Check sheet for the drawn part. Datum: minimum x, y, z corner. Units: mm. Coordinates: 2 decimals unless noted, no trailing zeros. Write each loop counter-clockwise with the first axis right and the second up, starting at its lowest first coordinate (ties: lowest second). Pieces come first, ordered by that corner, then holes. Notation, with made-up numbers: (-2.75, 44.5) - (6.25, 44.5) arc R9 ccw to (6.25, 57.5) - close; hole circle Ø2 at (39, 5.25). An arc over 180 degrees is marked (long way). Write each question's results on one line, items separated by ' | '.
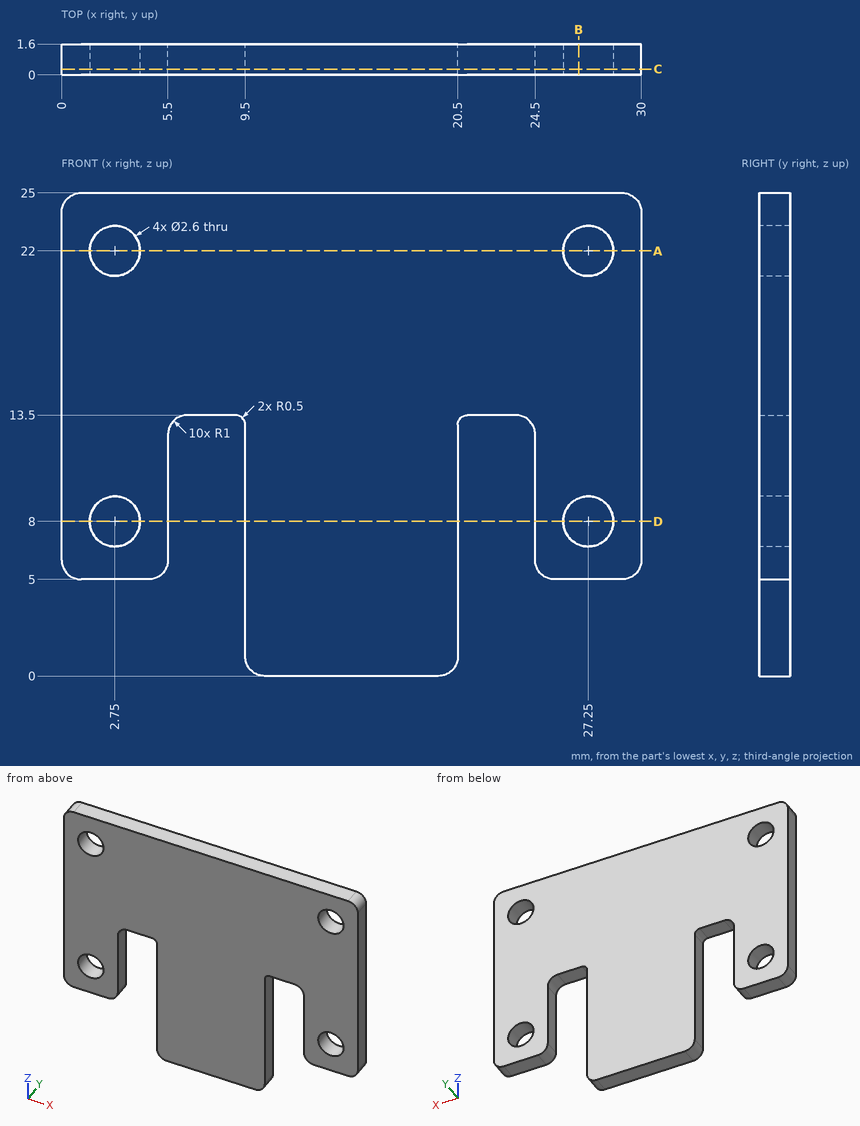
1. Sectioned sample at B-B (x = 26.75). Record the cut outline in (y, z).
Values follow:
outline: (0, 5) - (1.6, 5) - (1.6, 6.8) - (0, 6.8) - close; (0, 9.2) - (1.6, 9.2) - (1.6, 20.8) - (0, 20.8) - close; (0, 23.2) - (1.6, 23.2) - (1.6, 25) - (0, 25) - close
2. Sectioned sample at D-D (z = 8). Record the cut outline in (x, y), then the cut area to 3 significant figures.
Values follow:
outline: (0, 0) - (1.45, 0) - (1.45, 1.6) - (0, 1.6) - close; (4.05, 0) - (5.5, 0) - (5.5, 1.6) - (4.05, 1.6) - close; (9.5, 0) - (20.5, 0) - (20.5, 1.6) - (9.5, 1.6) - close; (24.5, 0) - (25.95, 0) - (25.95, 1.6) - (24.5, 1.6) - close; (28.55, 0) - (30, 0) - (30, 1.6) - (28.55, 1.6) - close | area: 26.9 mm^2
3. Sectioned sample at C-C (y = 0.3). Record the cut outline in (x, z), then the cut area to 3 significant figures.
Values follow:
outline: (0, 6) arc R1 ccw to (1, 5) - (4.5, 5) arc R1 ccw to (5.5, 6) - (5.5, 12.5) arc R1 cw to (6.5, 13.5) - (9, 13.5) arc R0.5 cw to (9.5, 13) - (9.5, 1) arc R1 ccw to (10.5, 0) - (19.5, 0) arc R1 ccw to (20.5, 1) - (20.5, 13) arc R0.5 cw to (21, 13.5) - (23.5, 13.5) arc R1 cw to (24.5, 12.5) - (24.5, 6) arc R1 ccw to (25.5, 5) - (29, 5) arc R1 ccw to (30, 6) - (30, 24) arc R1 ccw to (29, 25) - (1, 25) arc R1 ccw to (0, 24) - close; hole circle Ø2.6 at (2.75, 8); hole circle Ø2.6 at (2.75, 22); hole circle Ø2.6 at (27.25, 8); hole circle Ø2.6 at (27.25, 22) | area: 565 mm^2
4. Go/stop test with flat-tipped pins: pin 1 (3.5 mm diameter, centred on x = 2.75, z = 22, fed in from -Y); pin 2 (2.5 mm diameter, centred on x = 27.25, z = 8, fed in from -Y); pin 3 (0.8 mm diameter, centred on x = 22, y = 1, fed in from -Z). Record where each tip stops, or that it passes through.
Values follow:
pin 1: stops at y = 0 | pin 2: passes through | pin 3: stops at z = 13.5
5. Sectioned sample at A-A (z = 22). Record the cut outline in (x, y), then the cut area to 3 significant figures.
Values follow:
outline: (0, 0) - (1.45, 0) - (1.45, 1.6) - (0, 1.6) - close; (4.05, 0) - (25.95, 0) - (25.95, 1.6) - (4.05, 1.6) - close; (28.55, 0) - (30, 0) - (30, 1.6) - (28.55, 1.6) - close | area: 39.7 mm^2
6. Material ranges on L1, parallel to Z at x = 27.25, y = 0.7; L2, parallel to X at y = 0.5, z = 11.25; L3, parallel to X at y = 0.9, z = 8, recorded low to high. Write a range as [from, to].
Values follow:
L1: z = [5, 6.7], [9.3, 20.7], [23.3, 25] | L2: x = [0, 5.5], [9.5, 20.5], [24.5, 30] | L3: x = [0, 1.45], [4.05, 5.5], [9.5, 20.5], [24.5, 25.95], [28.55, 30]
